Can you work these out from the model? Positions are in its coordinate system, mm. Face numbers are marked on the shaded views. A direction names the side the tool comes from. Coordinates: 2 decimals unless noted, no trailing zeros. Order: outer loops, then holes, each group sorted by start corner. A loop starts at its lowest first (then second) coordinate and runs counter-clockwise, first axis right, second up. Notation, with made-up numbers: (49.5, 79.25) -> (71.5, 79.25) arc R22 ccw to (71.5, 98.25) -> close; hole circle Ø11 at (40, 34.25). An arc over 180 degrees is marked (long way). Answer in a Markdown table with one row per item.
```python
from build123d import *

# Parameters (mm, degrees)
BOSS_EXTRUDE1_DEPTH = 31.75
SKETCH19_W          = 15.860402013
SKETCH19_H          = 31.75
BOSS_EXTRUDE7_DEPTH = 2
SKETCH23_W          = 15.860402013
SKETCH23_H          = 4
BOSS_EXTRUDE8_DEPTH = 25
SKETCH24_R          = 1.27
CUT_EXTRUDE1_DEPTH  = 9


with BuildPart() as part:
    # Sketch2 → Boss-Extrude1 (new body)
    with BuildSketch(Plane.XY):
        with BuildLine():
            Line((-50.375618534, 45.609862895), (-50.351188886, 46.309436474))
            ThreePointArc((-50.351188886, 46.309436474), (-50.565618587, 46.88295476), (-51.12278195, 47.136868733))
            Line((-51.12278195, 47.136868733), (-55.780902554, 47.299533889))
            Line((-55.780902554, 47.299533889), (-47.850701548, 47.299533889))
            Line((-47.850701548, 47.299533889), (-47.850701548, 40.900752235))
            Line((-47.850701548, 40.900752235), (-48.952946324, 40.900752235))
            ThreePointArc((-48.952946324, 40.900752235), (-50.100996621, 41.129113637), (-51.074266668, 41.779431891))
            Line((-51.074266668, 41.779431891), (-53.375146928, 44.080312152))
            ThreePointArc((-53.375146928, 44.080312152), (-53.536830204, 44.931922499), (-52.803734096, 45.394471696))
            Line((-52.803734096, 45.394471696), (-50.685905631, 45.320515496))
            ThreePointArc((-50.685905631, 45.320515496), (-50.470836274, 45.400926634), (-50.375618534, 45.609862895))
        make_face()
    boss_extrude1 = extrude(amount=BOSS_EXTRUDE1_DEPTH)

    # Mirror2: Boss-Extrude1 across plane
    add(boss_extrude1.mirror(Plane(origin=(-47.850701548, 40.900752235, 31.75), x_dir=(0, 0, 1), z_dir=(-1, 0, 0))))

    # Sketch19 → Boss-Extrude7 (add)
    with BuildSketch(Plane(origin=(0, 47.299533889, 0), x_dir=(1, 0, 0), z_dir=(0, 1, 0))):
        with Locations((-47.850701548, -15.875)):
            Rectangle(SKETCH19_W, SKETCH19_H)
    extrude(amount=BOSS_EXTRUDE7_DEPTH)

    # Sketch23 → Boss-Extrude8 (add)
    with BuildSketch(Plane(origin=(0, 49.299533889, 0), x_dir=(1, 0, 0), z_dir=(0, 1, 0))):
        with Locations((-47.850701548, -25.75)):
            Rectangle(SKETCH23_W, SKETCH23_H)
    extrude(amount=BOSS_EXTRUDE8_DEPTH)

    # Sketch24 → Cut-Extrude1 (cut, through all)
    with BuildSketch(Plane(origin=(0, 0, 23.75), x_dir=(-1, 0, 0), z_dir=(0, 0, -1))):
        with Locations((47.850701548, 67.949533889)):
            Circle(SKETCH24_R)
    extrude(amount=-CUT_EXTRUDE1_DEPTH, mode=Mode.SUBTRACT)


solid = part.part
```
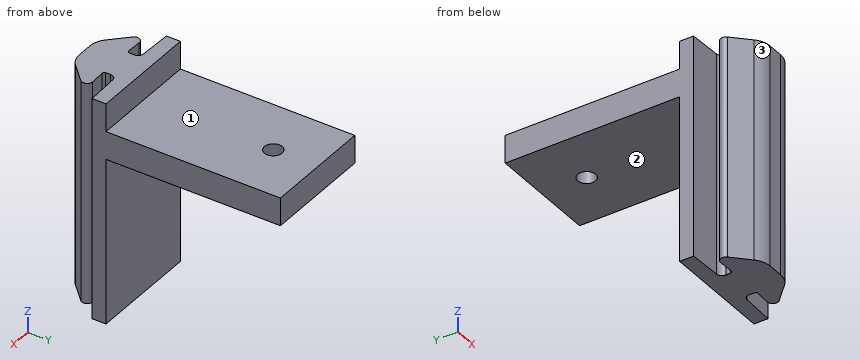
(1) Suppose I cut it at C-C (z = 21). Please give me the cut outline in (x, y).
Response values:
| item | result |
|---|---|
| outline | (-55.78, 47.3) -> (-51.12, 47.14) arc R0.8 cw to (-50.35, 46.31) -> (-50.38, 45.61) arc R0.3 cw to (-50.69, 45.32) -> (-52.8, 45.39) arc R0.77 ccw to (-53.38, 44.08) -> (-51.07, 41.78) arc R3 ccw to (-48.95, 40.9) -> (-46.75, 40.9) arc R3 ccw to (-44.63, 41.78) -> (-42.33, 44.08) arc R0.77 ccw to (-42.9, 45.39) -> (-45.02, 45.32) arc R0.3 cw to (-45.33, 45.61) -> (-45.35, 46.31) arc R0.8 cw to (-44.58, 47.14) -> (-39.92, 47.3) -> (-39.92, 49.3) -> (-55.78, 49.3) -> close |
(2) Suppose I cut it at A-A (z = 26.5). Please give me the cut outline in (x, y), and give its area (3 significant figures).
Response values:
| item | result |
|---|---|
| outline | (-55.78, 47.3) -> (-51.12, 47.14) arc R0.8 cw to (-50.35, 46.31) -> (-50.38, 45.61) arc R0.3 cw to (-50.69, 45.32) -> (-52.8, 45.39) arc R0.77 ccw to (-53.38, 44.08) -> (-51.07, 41.78) arc R3 ccw to (-48.95, 40.9) -> (-46.75, 40.9) arc R3 ccw to (-44.63, 41.78) -> (-42.33, 44.08) arc R0.77 ccw to (-42.9, 45.39) -> (-45.02, 45.32) arc R0.3 cw to (-45.33, 45.61) -> (-45.35, 46.31) arc R0.8 cw to (-44.58, 47.14) -> (-39.92, 47.3) -> (-39.92, 74.3) -> (-55.78, 74.3) -> close; hole circle Ø2.54 at (-47.85, 67.95) |
| area | 473 mm2 |
(3) Suppose I cut it at D-D (x = -54.5). Please give me the cut outline in (y, z).
Response values:
| item | result |
|---|---|
| outline | (47.25, 0) -> (49.3, 0) -> (49.3, 23.75) -> (74.3, 23.75) -> (74.3, 27.75) -> (49.3, 27.75) -> (49.3, 31.75) -> (47.25, 31.75) -> close |
(4) Suppose I cut it at B-B (x = -43.5). Please give me the cut outline in (y, z).
Response values:
| item | result |
|---|---|
| outline | (42.91, 0) -> (45.37, 0) -> (45.37, 31.75) -> (42.91, 31.75) -> close; (47.17, 0) -> (49.3, 0) -> (49.3, 23.75) -> (74.3, 23.75) -> (74.3, 27.75) -> (49.3, 27.75) -> (49.3, 31.75) -> (47.17, 31.75) -> close |
(5) On a 3-axis mill with a long thin cutter (end or side, diameter ignored), from which of +Z, -Z, +X, -X, +Y, -Y can I reach the whole of each face in a straight line? I mean the marked faces 1, 2 and 3. Say none if no direction works.
Response values:
| item | result |
|---|---|
| face 1 | +Z, +X, -X, +Y |
| face 2 | -Z, +X, -X, +Y |
| face 3 | +Z, -Z, -X, -Y |
(6) I need wall thicknesses on line 1 (Y direction, x = -47.25, z = 17); line 2 (Z direction, x = -49.75, y = 55); line 3 (Y direction, x = -42.25, z = 2). Which ranges of each line are inside material? Lowest first, please. Write a range as [from, to].
Response values:
| item | result |
|---|---|
| line 1 | [40.9, 49.3] |
| line 2 | [23.75, 27.75] |
| line 3 | [44.17, 45.08], [47.22, 49.3] |
(7) Will these pins go through, and if not, where does the flat tip stop? pin 1 Ø8 at (x, y) = (-51.5, 63) entering from +Z; pin 2 Ø1 at (x, z) = (-51.5, 22.5) entering from +Y; pin 3 Ø3.5 at (x, y) = (-47.85, 67.95) entering from -Z.
Response values:
| item | result |
|---|---|
| pin 1 | z = 27.75 |
| pin 2 | y = 49.3 |
| pin 3 | z = 23.75 |
